Geometry: final body of the model. Coordinates: model frame, mm. Round coordinates to 2 decimals unless told otherwise and drop trailing zeros. Loops run counter-clockwise (first coordinate to the right, second up) from the corner with the lowest first, then second, coordinate; pieces in that order, holes last. Notation, with made-up numbers: M 23.5,74 L 66.5,74 A17 cw 66.5,79 Z; hole C 14.5,20 d5. An arc over 180 degrees is marked long. Write each question's results on one line, items separated by ' | '.
```python
from build123d import *

# Parameters (mm, degrees)
F0_R     = 48.925
F0_R_2   = 35.2
F1_DEPTH = 2.5
F3_D     = 6.5


with BuildPart() as f1:
    # F0 (on Front) → F1 (new body)
    with BuildSketch(Plane.XZ):
        Circle(F0_R)
        Circle(F0_R_2, mode=Mode.SUBTRACT)
    extrude(amount=-F1_DEPTH)

    # F3 (through all)
    with Locations(Plane.XZ):
        with Locations((0, 42.5), (-36.80608, -21.25), (36.80608, -21.25)):
            Hole(F3_D / 2)


solid = f1.part
```
1. Section B-B (x = 6). Output: boundary loops of the cut face in (y, z), then the cut area to 3 significant figures.
Answer key:
outline: M 0,-48.56 L 2.5,-48.56 L 2.5,-34.68 L 0,-34.68 Z; M 0,34.68 L 2.5,34.68 L 2.5,48.56 L 0,48.56 Z | area: 69.4 mm²
2. Pin query (flat end, axial travel): P1, Ø10, axis at x = 25.5, z = -8, coming from the +Y side. Return the tip coordinate at first contact, or that it passes through.
Answer key:
P1: passes through
3. Section A-A (z = 0). Output: boundary loops of the cut face in (x, y) (3 decimals), then the cut area to 3 significant figures.
Answer key:
outline: M -48.925,0 L -35.2,0 L -35.2,2.5 L -48.925,2.5 Z; M 35.2,0 L 48.925,0 L 48.925,2.5 L 35.2,2.5 Z | area: 68.6 mm²
4. Section D-D (z = -21.25). Output: boundary loops of the cut face in (x, y), then the cut area to 3 significant figures.
Answer key:
outline: M -44.07,0 L -40.06,0 L -40.06,2.5 L -44.07,2.5 Z; M -33.56,0 L -28.06,0 L -28.06,2.5 L -33.56,2.5 Z; M 28.06,0 L 33.56,0 L 33.56,2.5 L 28.06,2.5 Z; M 40.06,0 L 44.07,0 L 44.07,2.5 L 40.06,2.5 Z | area: 47.5 mm²
5. Section C-C (y = 1.35). Output: boundary loops of the cut face in (x, z) (3 decimals), then the cut area to 3 significant figures.
Answer key:
outline: C 0,0 d97.85; hole C -36.806,-21.25 d6.5; hole C 0,0 d70.4; hole C 0,42.5 d6.5; hole C 36.806,-21.25 d6.5 | area: 3,530 mm²
6. Ray query, probe 1 along Z at (x, y) = (0, 1.05) (3 decimals); probe 2 along X at (y, z) = (0.95, -0.5); probe 3 along Z at (x, y) = (-12, 2.2). Return the intervals inside material, ascending.
Answer key:
probe 1: z = -48.925 to -35.2, 35.2 to 39.25, 45.75 to 48.925 | probe 2: x = -48.92 to -35.2, 35.2 to 48.92 | probe 3: z = -47.43 to -33.09, 33.09 to 47.43
7. Draft query along X for faces 1 (the face through (22, 2.5, 29)), 2 (the face through (-10.61, 1.23, -47.76)), 3 (the face through (-33.56, 1.27, -21.11)). Return one class per face: pulls with the +X half, pulls with the -X half, needs draft (parallel to the pull), parting line crosses it, or undercut.
Answer key:
face 1: needs draft | face 2: parting line crosses it | face 3: undercut
